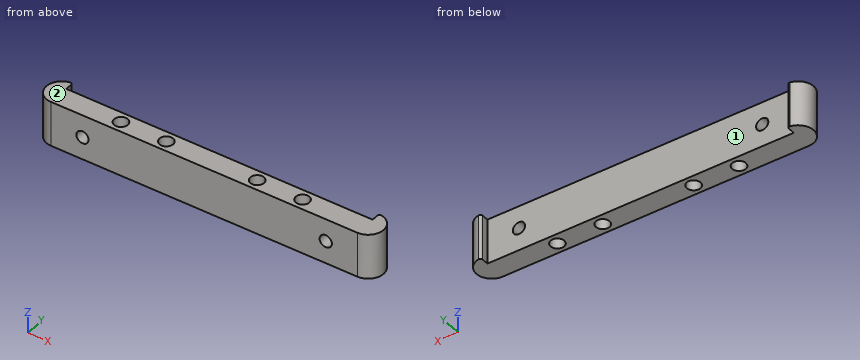
```python
from build123d import *

# Parameters (mm, degrees)
SKETCH1_R           = 2.413
BOSS_EXTRUDE1_DEPTH = 15.8242
SKETCH3_R           = 2.159
CUT_EXTRUDE1_DEPTH  = 7.62
FILLET1_R           = 0.762


with BuildPart() as part:
    # Sketch1 → Boss-Extrude1 (new body)
    with BuildSketch(Plane.XY):
        with BuildLine():
            Line((0, 7.62), (107.95, 7.62))
            Line((107.95, 7.62), (107.95, 10.8204))
            ThreePointArc((107.95, 10.8204), (113.3602, 5.4102), (107.95, 0))
            Line((107.95, 0), (0, 0))
            ThreePointArc((0, 0), (-5.4102, 5.4102), (0, 10.8204))
            Line((0, 10.8204), (0, 7.62))
        make_face()
        with Locations((21.971, 3.81)):
            Circle(SKETCH1_R, mode=Mode.SUBTRACT)
        with Locations((37.973, 3.81)):
            Circle(SKETCH1_R, mode=Mode.SUBTRACT)
        with Locations((69.977, 3.81)):
            Circle(SKETCH1_R, mode=Mode.SUBTRACT)
        with Locations((85.979, 3.81)):
            Circle(SKETCH1_R, mode=Mode.SUBTRACT)
    extrude(amount=BOSS_EXTRUDE1_DEPTH)

    # Sketch3 → Cut-Extrude1 (cut)
    with BuildSketch(Plane(origin=(0, 7.62, 0), x_dir=(1, 0, 0), z_dir=(0, 1, 0))):
        with Locations((96.8375, -7.9121)):
            Circle(SKETCH3_R)
        with Locations((11.1125, -7.9121)):
            Circle(SKETCH3_R)
    extrude(amount=-CUT_EXTRUDE1_DEPTH, mode=Mode.SUBTRACT)

    # Fillet1
    fillet1_edges = [part.edges().sort_by_distance(p)[0] for p in [
        (0, 10.8204, 7.9121),
        (107.95, 10.8204, 7.9121),
    ]]
    fillet(fillet1_edges, radius=FILLET1_R)


solid = part.part
```
The listing builds one solid part. Answer for the finished solid, in the listing's coordinates (mm). Face numbers are marked on the shaded views. A direction names the side the tool comes from. Round coordinates to 2 decimals unless told otherwise and drop trailing zeros. Order: outer loops, then holes, each group sorted by start corner. A loop starts at its lowest first (then second) coordinate and runs counter-clockwise, first axis right, second up. Notation, with made-up numbers: (31, 48) -> (60, 48) arc R31 cw to (60, 74) -> close; hole circle Ø1 at (20.25, 86.5). An arc over 180 degrees is marked (long way). Answer as CSV lines item,"result". Start each with the question number.
(1) The part is cut by section D-D (y = 8.75). Determine the outline of the cut face in (x, z), then the cut area to 3 significant figures.
(2) The part is cut by section C-C (x = 71). Determine the outline of the cut face in (y, z), then the cut area to 3 significant figures.
(3) The part is cut by section B-B (y = 3.81). Determine the outline of the cut face in (x, z).
(4) The part is cut by section A-A (z = 11.75). Determine the outline of the cut face in (x, y), then the cut area to 3 significant figures.
(5) Flat-ended cylindrical pins translate along their axes: pin 1 Ø5 at (y, z) = (4, 12.5) entering from +X; pin 2 Ø1 at (y, z) = (6.5, 12) entering from +X; pin 3 Ø1.5 at (x, z) = (92.5, 9) entering from +Y; pin 4 Ø3 at (x, y) = (85.979, 3.81) entering from +Z. Find the tip coordinate at first contact, or state that the pin passes through.
(6) Find the intervals of material crossed by probe 1 along X at (y, z) = (5.25, 12.5); probe 2 along X at (y, z) = (4, 14.25); probe 3 along Y at (x, z) = (17, 6.25), in increasing order. Write a range as from..to.
(7) A tool of negligible diameter and unlimited length cuts with its end or side. For the marked faces 1 and 2, from which of +Z, -Z, +X, -X, +Y, -Y can it reach the whole face along a straight path? Write none if from no direction.
Evaluation:
1,outline,"(-4.26, 0) -> (0, 0) -> (0, 15.82) -> (-4.26, 15.82) -> close; (107.95, 0) -> (112.21, 0) -> (112.21, 15.82) -> (107.95, 15.82) -> close"
1,area,"135 mm²"
2,outline,"(0, 0) -> (1.62, 0) -> (1.62, 15.82) -> (0, 15.82) -> close; (6, 0) -> (7.62, 0) -> (7.62, 15.82) -> (6, 15.82) -> close"
2,area,"51.4 mm²"
3,outline,"(-5.17, 0) -> (19.56, 0) -> (19.56, 15.82) -> (-5.17, 15.82) -> close; (24.38, 0) -> (35.56, 0) -> (35.56, 15.82) -> (24.38, 15.82) -> close; (40.39, 0) -> (67.56, 0) -> (67.56, 15.82) -> (40.39, 15.82) -> close; (72.39, 0) -> (83.57, 0) -> (83.57, 15.82) -> (72.39, 15.82) -> close; (88.39, 0) -> (113.12, 0) -> (113.12, 15.82) -> (88.39, 15.82) -> close; hole circle Ø4.32 at (11.11, 7.91); hole circle Ø4.32 at (96.84, 7.91)"
4,outline,"(-0.89, 10.75) arc R5.41 ccw to (0, 0) -> (107.95, 0) arc R5.41 ccw to (108.84, 10.75) arc R0.76 ccw to (107.95, 10) -> (107.95, 7.62) -> (0, 7.62) -> (0, 10) arc R0.76 ccw to start; hole circle Ø4.83 at (21.97, 3.81); hole circle Ø4.83 at (37.97, 3.81); hole circle Ø4.83 at (69.98, 3.81); hole circle Ø4.83 at (85.98, 3.81)"
4,area,"841 mm²"
5,pin 1,"x = 113.36"
5,pin 2,"x = 113.33"
5,pin 3,"y = 7.62"
5,pin 4,"through"
6,probe 1,"-5.41..20.03, 23.91..36.04, 39.91..68.04, 71.91..84.04, 87.92..113.36"
6,probe 2,"-5.22..19.57, 24.38..35.57, 40.38..67.57, 72.38..83.57, 88.38..113.17"
6,probe 3,"0..7.62"
7,face 1,"+Z, -Z, +Y"
7,face 2,"+Z, +X, -X, +Y, -Y"
